Source: CAD feature listing. Evaluate the final solid. Frame: model axes, mm. A direction names the side the tool comes from. Round coordinates to 2 decimals unless told otherwise and drop trailing zeros. Order: outer loops, then holes, each group sorted by start corner. A loop starts at its lowest first (then second) coordinate and runs counter-clockwise, first axis right, second up. Notation, with made-up numbers: M 32.5,-35.75 L 45.5,-35.75 A27 ccw 45.5,-15.75 Z; hole C 71,53.25 d2. An arc over 180 degrees is marked long. Use one line per item in the form item = value. Start each with the question number.
Q1. Material intervals for probe 1 along Y at (x, z) = (2.5, 9.5); probe 2 along X at (y, z) = (15.5, 1.75); probe 3 along X at (y, z) = (-3, 6.75), sorted ascending.
Q2. Section C-C (x = 0). Return the cut outline in (y, z).
Q3. Reachability of faces 1 (the cylindrical face through (-11.57, -20.97, 4.93)), 2 (the cylindrical face through (-13.15, 23.97, 4.93)), 3 (the cylindrical face through (13.99, 6.02, 4.93)) from +Z, -Z, +X, -X, +Y, -Y: full face, straight path, thin tool, end or side. Return the list, or none.
Q4. Section B-B (y = 6). Return the cut outline in (x, z), plus the area to 3 significant figures.
Q5. Pull-direction query (Y, two-part tool) for faces 4 (the flat face through (-5.3, -10.2, 0)), 5 (the cylindrical face through (12.357, 29.74, 4.93)), 6 (the cylindrical face through (-8.09, -13.72, 4.93)), 7 (the cylindrical face through (17.303, -24.909, 4.93)); classes: pulls with the +Y half, pulls with the -Y half, needs draft (parallel to the pull), parting line crosses it, or undercut.
Q6. Section A-A (x = 24). Return the cut outline in (y, z).
Q7. Contact query for flat-ended pins moving along their axis: pin 1 (6 mm diameter, centred on y = -16.5, z = 5.5, fed in from -X); pin 2 (1.5 mm diameter, centred on x = 15, z = 6, fed in from +Y). Output: stop coordinate, or through.
Q8. Section D-D (z = 7.75). Give the number of separate pieces and of enclosed holes in the cut face, plus the area to 3 significant figures.
from build123d import *

# Parameters (mm, degrees)
F0_R     = 11.2
F1_DEPTH = 10


with BuildPart() as f1:
    # F0 (on Top) → F1 (new body)
    with BuildSketch(Plane.XY):
        with BuildLine():
            ThreePointArc((-3.260381, 12.308222), (-4.08829, 12.548299), (-4.898764, 12.841902))
            ThreePointArc((-4.898764, 12.841902), (-7.873837, 13.885182), (-10.533641, 15.577793))
            ThreePointArc((-10.533641, 15.577793), (-10.432312, 14.889978), (-10.350403, 14.199581))
            ThreePointArc((-10.350403, 14.199581), (-6.9123, 12.853141), (-3.260381, 12.308222))
        make_face()
        with BuildLine():
            ThreePointArc((-10.999331, 17.801648), (-11.517235, 18.649945), (-11.969844, 19.534805))
            ThreePointArc((-11.969844, 19.534805), (-12.253411, 8.962243), (-18.075311, 0.132465))
            ThreePointArc((-18.075311, 0.132465), (-16.04011, -0.642041), (-14.159937, -1.740609))
            ThreePointArc((-14.159937, -1.740609), (-11.356021, 4.229127), (-10.233904, 10.7284))
            ThreePointArc((-10.233904, 10.7284), (-10.217244, 11.71927), (-10.240391, 12.710009))
            ThreePointArc((-10.240391, 12.710009), (-10.284122, 13.455628), (-10.350403, 14.199581))
            ThreePointArc((-10.350403, 14.199581), (-10.432312, 14.889978), (-10.533641, 15.577793))
            ThreePointArc((-10.533641, 15.577793), (-10.740872, 16.695084), (-10.999331, 17.801648))
        make_face()
        with BuildLine():
            ThreePointArc((-25.815076, 0.0045), (-27.634187, -0.740376), (-29.322511, -1.747138))
            ThreePointArc((-29.322511, -1.747138), (-30.235928, -2.541319), (-31.167579, -3.314027))
            ThreePointArc((-31.167579, -3.314027), (-31.944836, -4.181143), (-32.642648, -5.113387))
            Line((-32.642648, -5.113387), (-33.685691, -6.940824))
            ThreePointArc((-33.685691, -6.940824), (-30.831382, -22.116455), (-15.530856, -24.199898))
            ThreePointArc((-15.530856, -24.199898), (-14.161107, -23.359441), (-12.903641, -22.358761))
            ThreePointArc((-12.903641, -22.358761), (-12.582952, -22.041715), (-12.254476, -21.732744))
            ThreePointArc((-12.254476, -21.732744), (-11.562129, -20.959176), (-10.932716, -20.133592))
            ThreePointArc((-10.932716, -20.133592), (-10.392709, -19.299191), (-9.917014, -18.426525))
            ThreePointArc((-9.917014, -18.426525), (-8.886316, -15.568046), (-8.536572, -12.549615))
            ThreePointArc((-8.536572, -12.549615), (-8.57048, -11.604081), (-8.672031, -10.663405))
            ThreePointArc((-8.672031, -10.663405), (-8.823001, -9.814713), (-9.029042, -8.977684))
            ThreePointArc((-9.029042, -8.977684), (-9.262483, -8.232543), (-9.539575, -7.50251))
            ThreePointArc((-9.539575, -7.50251), (-9.896819, -6.7135), (-10.305036, -5.949615))
            ThreePointArc((-10.305036, -5.949615), (-12.002273, -3.634267), (-14.159937, -1.740609))
            ThreePointArc((-14.159937, -1.740609), (-16.04011, -0.642041), (-18.075311, 0.132465))
            ThreePointArc((-18.075311, 0.132465), (-21.503799, 0.648332), (-24.948347, 0.253685))
            ThreePointArc((-24.948347, 0.253685), (-25.380161, 0.123701), (-25.815076, 0.0045))
        make_face()
        with Locations((-21.736572, -12.549615)):
            Circle(F0_R, mode=Mode.SUBTRACT)
        with BuildLine():
            ThreePointArc((-10.240391, 12.710009), (-10.217244, 11.71927), (-10.233904, 10.7284))
            ThreePointArc((-10.233904, 10.7284), (-5.051167, 10.738809), (0, 11.899231))
            ThreePointArc((0, 11.899231), (-0.865652, 11.927646), (-1.727577, 12.012769))
            ThreePointArc((-1.727577, 12.012769), (-6.049129, 11.566016), (-10.240391, 12.710009))
        make_face()
        with BuildLine():
            ThreePointArc((9.152374, 15.587446), (7.464031, 14.212163), (5.572557, 13.13317))
            ThreePointArc((5.572557, 13.13317), (9.340542, 7.720039), (14.408019, 3.498621))
            ThreePointArc((14.408019, 3.498621), (15.257807, 2.988758), (16.127386, 2.513434))
            ThreePointArc((16.127386, 2.513434), (16.794976, 2.178497), (17.472399, 1.863922))
            ThreePointArc((17.472399, 1.863922), (18.111255, 1.589658), (18.757585, 1.333505))
            ThreePointArc((18.757585, 1.333505), (19.828803, 0.954326), (20.916345, 0.624876))
            ThreePointArc((20.916345, 0.624876), (21.909944, 0.649246), (22.90256, 0.598786))
            ThreePointArc((22.90256, 0.598786), (13.888235, 6.130644), (9.152374, 15.587446))
        make_face()
        with BuildLine():
            ThreePointArc((-10.233904, 10.7284), (-11.356021, 4.229127), (-14.159937, -1.740609))
            ThreePointArc((-14.159937, -1.740609), (-12.002273, -3.634267), (-10.305036, -5.949615))
            ThreePointArc((-10.305036, -5.949615), (-6.774498, -9.743843), (-4.174115, -14.227021))
            ThreePointArc((-4.174115, -14.227021), (2.015479, -11.949166), (8.587381, -11.392561))
            ThreePointArc((8.587381, -11.392561), (9.148504, -8.57714), (10.305036, -5.949615))
            ThreePointArc((10.305036, -5.949615), (11.825665, -0.994965), (14.408019, 3.498621))
            ThreePointArc((14.408019, 3.498621), (9.340542, 7.720039), (5.572557, 13.13317))
            ThreePointArc((5.572557, 13.13317), (2.853769, 12.211407), (0, 11.899231))
            ThreePointArc((0, 11.899231), (-5.051167, 10.738809), (-10.233904, 10.7284))
        make_face()
        Circle(F0_R, mode=Mode.SUBTRACT)
        with BuildLine():
            ThreePointArc((8.587381, -11.392561), (2.015479, -11.949166), (-4.174115, -14.227021))
            ThreePointArc((-4.174115, -14.227021), (-5.040564, -14.708027), (-5.886995, -15.223443))
            ThreePointArc((-5.886995, -15.223443), (-6.510854, -15.634125), (-7.121996, -16.063503))
            ThreePointArc((-7.121996, -16.063503), (-7.678943, -16.479636), (-8.223944, -16.911297))
            ThreePointArc((-8.223944, -16.911297), (-9.087931, -17.64941), (-9.917014, -18.426525))
            ThreePointArc((-9.917014, -18.426525), (-10.392709, -19.299191), (-10.932716, -20.133592))
            ThreePointArc((-10.932716, -20.133592), (-1.634824, -15.092886), (8.922937, -15.719911))
            ThreePointArc((8.922937, -15.719911), (8.576079, -13.570122), (8.587381, -11.392561))
        make_face()
        with BuildLine():
            ThreePointArc((-7.121996, -16.063503), (-7.674996, -12.412798), (-9.029042, -8.977684))
            ThreePointArc((-9.029042, -8.977684), (-8.823001, -9.814713), (-8.672031, -10.663405))
            ThreePointArc((-8.672031, -10.663405), (-8.088002, -13.761534), (-8.223944, -16.911297))
            ThreePointArc((-8.223944, -16.911297), (-7.678943, -16.479636), (-7.121996, -16.063503))
        make_face()
        with BuildLine():
            ThreePointArc((-4.174115, -14.227021), (-6.774498, -9.743843), (-10.305036, -5.949615))
            ThreePointArc((-10.305036, -5.949615), (-9.896819, -6.7135), (-9.539575, -7.50251))
            ThreePointArc((-9.539575, -7.50251), (-6.991899, -11.021707), (-5.886995, -15.223443))
            ThreePointArc((-5.886995, -15.223443), (-5.040564, -14.708027), (-4.174115, -14.227021))
        make_face()
        with BuildLine():
            ThreePointArc((12.289423, -3.330538), (12.911291, -2.733587), (13.570796, -2.178497))
            ThreePointArc((13.570796, -2.178497), (15.961839, -0.123648), (18.757585, 1.333505))
            ThreePointArc((18.757585, 1.333505), (18.111255, 1.589658), (17.472399, 1.863922))
            ThreePointArc((17.472399, 1.863922), (14.587297, -0.440343), (12.289423, -3.330538))
        make_face()
        with BuildLine():
            ThreePointArc((14.408019, 3.498621), (11.825665, -0.994965), (10.305036, -5.949615))
            ThreePointArc((10.305036, -5.949615), (10.76247, -5.214146), (11.267152, -4.510259))
            ThreePointArc((11.267152, -4.510259), (13.041028, -0.544309), (16.127386, 2.513434))
            ThreePointArc((16.127386, 2.513434), (15.257807, 2.988758), (14.408019, 3.498621))
        make_face()
        with BuildLine():
            ThreePointArc((34.936572, -12.549615), (33.279164, -6.145823), (28.723154, -1.350166))
            ThreePointArc((28.723154, -1.350166), (27.310423, -0.584158), (25.815076, 0.0045))
            ThreePointArc((25.815076, 0.0045), (25.380161, 0.123701), (24.948347, 0.253685))
            ThreePointArc((24.948347, 0.253685), (23.932244, 0.466491), (22.90256, 0.598786))
            ThreePointArc((22.90256, 0.598786), (21.909944, 0.649246), (20.916345, 0.624876))
            ThreePointArc((20.916345, 0.624876), (17.030003, -0.21721), (13.570796, -2.178497))
            ThreePointArc((13.570796, -2.178497), (12.911291, -2.733587), (12.289423, -3.330538))
            ThreePointArc((12.289423, -3.330538), (11.760833, -3.905274), (11.267152, -4.510259))
            ThreePointArc((11.267152, -4.510259), (10.76247, -5.214146), (10.305036, -5.949615))
            ThreePointArc((10.305036, -5.949615), (9.148504, -8.57714), (8.587381, -11.392561))
            ThreePointArc((8.587381, -11.392561), (8.576079, -13.570122), (8.922937, -15.719911))
            ThreePointArc((8.922937, -15.719911), (10.190428, -18.947002), (12.254476, -21.732744))
            ThreePointArc((12.254476, -21.732744), (12.582952, -22.041715), (12.903641, -22.358761))
            ThreePointArc((12.903641, -22.358761), (14.458278, -23.56172), (16.174322, -24.520471))
            ThreePointArc((16.174322, -24.520471), (17.31881, -24.914422), (18.453821, -25.334902))
            ThreePointArc((18.453821, -25.334902), (19.593394, -25.574468), (20.749647, -25.712669))
            Line((20.749647, -25.712669), (22.853775, -25.702252))
            ThreePointArc((22.853775, -25.702252), (31.457351, -21.479703), (34.936572, -12.549615))
        make_face()
        with Locations((21.736572, -12.549615)):
            Circle(F0_R, mode=Mode.SUBTRACT)
        with BuildLine():
            ThreePointArc((10.831916, 32.643076), (-3.737721, 37.758988), (-13.192299, 25.550065))
            ThreePointArc((-13.192299, 25.550065), (-13.149316, 23.943599), (-12.911435, 22.354261))
            ThreePointArc((-12.911435, 22.354261), (-12.797209, 21.918014), (-12.693871, 21.479059))
            ThreePointArc((-12.693871, 21.479059), (-12.370115, 20.492686), (-11.969844, 19.534805))
            ThreePointArc((-11.969844, 19.534805), (-11.517235, 18.649945), (-10.999331, 17.801648))
            ThreePointArc((-10.999331, 17.801648), (-8.326892, 14.857021), (-4.898764, 12.841902))
            ThreePointArc((-4.898764, 12.841902), (-4.08829, 12.548299), (-3.260381, 12.308222))
            ThreePointArc((-3.260381, 12.308222), (-2.49835, 12.137817), (-1.727577, 12.012769))
            ThreePointArc((-1.727577, 12.012769), (-0.865652, 11.927646), (0, 11.899231))
            ThreePointArc((0, 11.899231), (2.853769, 12.211407), (5.572557, 13.13317))
            ThreePointArc((5.572557, 13.13317), (7.464031, 14.212163), (9.152374, 15.587446))
            ThreePointArc((9.152374, 15.587446), (11.313372, 18.29867), (12.693871, 21.479059))
            ThreePointArc((12.693871, 21.479059), (12.797209, 21.918014), (12.911435, 22.354261))
            ThreePointArc((12.911435, 22.354261), (13.12766, 23.719183), (13.2, 25.099231))
            ThreePointArc((13.2, 25.099231), (13.187041, 25.683994), (13.14819, 26.267609))
            ThreePointArc((13.14819, 26.267609), (12.917117, 27.455741), (12.713758, 28.648929))
            ThreePointArc((12.713758, 28.648929), (12.351442, 29.755611), (11.893001, 30.826056))
            Line((11.893001, 30.826056), (10.831916, 32.643076))
        make_face()
        with Locations((0, 25.099231)):
            Circle(F0_R, mode=Mode.SUBTRACT)
    extrude(amount=F1_DEPTH)


solid = f1.part
Results list:
q1.probe_1 = -14.63 to -10.92, 10.92 to 14.18, 36.02 to 38.06
q1.probe_2 = -11.38 to -10.44, -9.06 to -5.77, 5.77 to 9.17
q1.probe_3 = -30.78 to -27.59, -15.88 to -10.79, 10.79 to 11.74, 12.5 to 15.88, 27.59 to 30.85
q2.outline = M -14.8,0 L -11.2,0 L -11.2,10 L -14.8,10 Z; M 11.2,0 L 13.9,0 L 13.9,10 L 11.2,10 Z; M 36.3,0 L 38.3,0 L 38.3,10 L 36.3,10 Z
q3.face_1 = +Z, -Z, -Y
q3.face_2 = +Z, -Z, -X
q3.face_3 = +Z, -Z, +X
q4.outline = M -13.46,0 L -9.46,0 L -9.46,10 L -13.46,10 Z; M 9.46,0 L 14.01,0 L 14.01,10 L 9.46,10 Z
q4.area = 85.6 mm2
q5.face_4 = needs draft
q5.face_5 = pulls with the +Y half
q5.face_6 = undercut
q5.face_7 = pulls with the -Y half
q6.outline = M -25.55,0 L -23.52,0 L -23.52,10 L -25.55,10 Z; M -1.58,0 L 0.45,0 L 0.45,10 L -1.58,10 Z
q7.pin_1 = -34.9
q7.pin_2 = 5.75
q8.separate_pieces = 1
q8.enclosed_holes = 10
q8.area = 734 mm2
